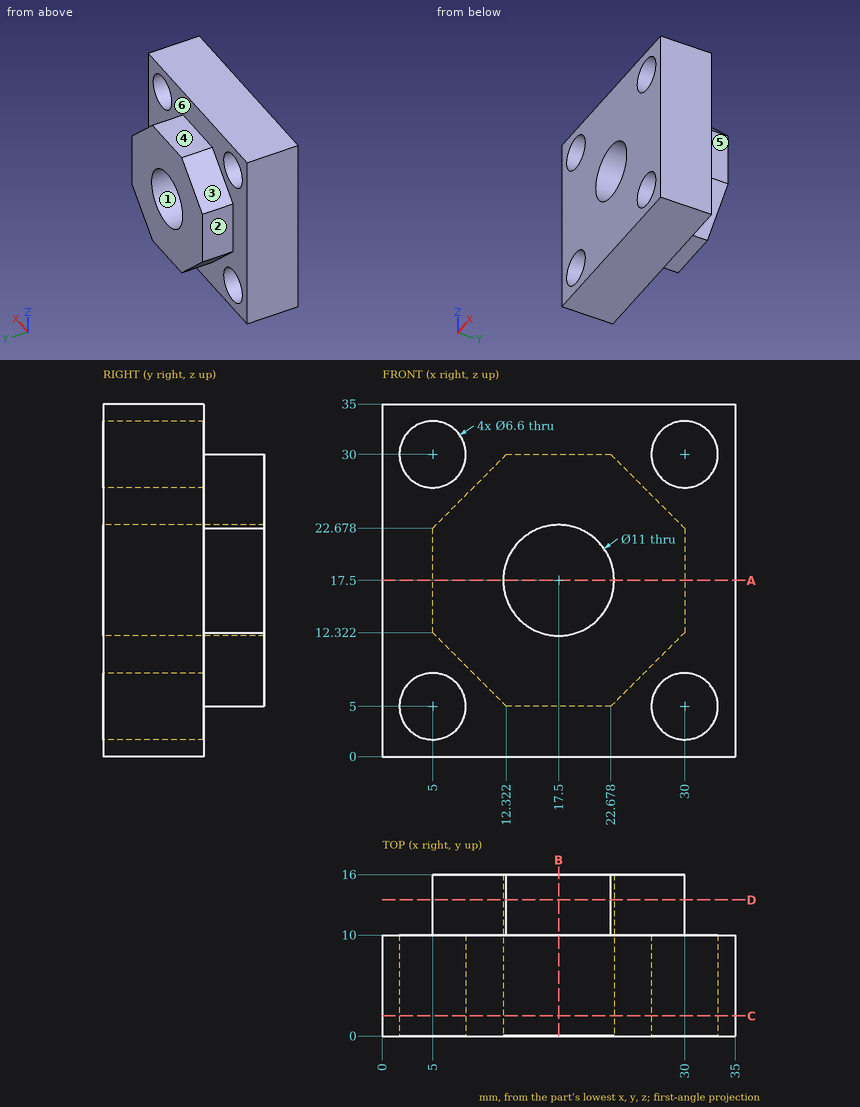
Geometry: see drawing. Coordinates: mm, zero at the bounding-box minimum. A direction names the side the tool comes from. Round coordinates to 2 decimals unless told otherwise and drop trailing zeros. Loops run counter-clockwise (first coordinate to the right, second up) from the corner with the lowest first, then second, coordinate; pieces in that order, holes last. Notation, with made-up numbers: (50, 0.5) -> (57, 0.5) arc R29 ccw to (57, 39.5) -> close; hole circle Ø10 at (-29.5, -15.5). An arc over 180 degrees is marked (long way). Use one line per item in the form item = value. Start each with the question number.
Item 1: Section query C-C on y = 2. Return the cut outline in (x, z), then the cut area to 3 significant figures.
Item 2: Mould query, pull axis Z, two halves, no side actions, for the marked faces 1, 2 and 3. Classes: pulls with the +Z half, pulls with the -Z half, needs draft (parallel to the pull), parting line crosses it, or undercut.
Item 3: Contact query for flat-ended pins moving along their axis: pin 1 Ø1.8 at (x, y) = (17.5, 14) entering from -Z; pin 2 Ø10 at (x, z) = (17.5, 17.5) entering from +Y; pin 3 Ø1.8 at (y, z) = (12, 18) entering from +X; pin 4 Ø3 at (x, y) = (16.5, 12.5) entering from +Z. Output: stop coordinate, or through.
Item 4: Section query D-D on y = 13.5. Return the cut outline in (x, z).
Item 5: Section query B-B on x = 17.5. Return the cut outline in (y, z).
Item 6: Material intervals for L1, parallel to Z at x = 5, y = 2.5; L2, parallel to X at y = 5.75, z = 17.5; L3, parallel to Z at x = 28.5, y = 7.5, sorted ascending. Write a range as from..to.
Item 7: Section query A-A on z = 17.5. Return the cut outline in (x, y).
Item 8: Set-up query: the marked faces 4, 5 and 6. Return all of +Z, -Z, +X, -X, +Y, -Y with unobstructed straight access to the full face (end or side cutting, diameter ignored); none if empty.
Ans:
q1.outline = (0, 0) -> (35, 0) -> (35, 35) -> (0, 35) -> close; hole circle Ø6.6 at (5, 5); hole circle Ø6.6 at (5, 30); hole circle Ø11 at (17.5, 17.5); hole circle Ø6.6 at (30, 5); hole circle Ø6.6 at (30, 30)
q1.area = 993 mm^2
q2.face_1 = undercut
q2.face_2 = needs draft
q2.face_3 = pulls with the +Z half
q3.pin_1 = 5
q3.pin_2 = through
q3.pin_3 = 30
q3.pin_4 = 30
q4.outline = (5, 12.32) -> (12.32, 5) -> (22.68, 5) -> (30, 12.32) -> (30, 22.68) -> (22.68, 30) -> (12.32, 30) -> (5, 22.68) -> close; hole circle Ø11 at (17.5, 17.5)
q5.outline = (0, 0) -> (10, 0) -> (10, 5) -> (16, 5) -> (16, 12) -> (0, 12) -> close; (0, 23) -> (16, 23) -> (16, 30) -> (10, 30) -> (10, 35) -> (0, 35) -> close
q6.L1 = 0..1.7, 8.3..26.7, 33.3..35
q6.L2 = 0..12, 23..35
q6.L3 = 0..2.06, 7.94..27.06, 32.94..35
q7.outline = (0, 0) -> (12, 0) -> (12, 16) -> (5, 16) -> (5, 10) -> (0, 10) -> close; (23, 0) -> (35, 0) -> (35, 10) -> (30, 10) -> (30, 16) -> (23, 16) -> close
q8.face_4 = +Z, +X, -X, +Y
q8.face_5 = +Z, -Z, +X, +Y
q8.face_6 = +Y
